Design review of the part built by this model. Coordinates are the model's own, in mm. Face numbers are marked on the shaded views. A direction names the side the tool comes from. Round coordinates to 2 decimals unless told otherwise and drop trailing zeros. Loops run counter-clockwise (first coordinate to the right, second up) from the corner with the lowest first, then second, coordinate; pieces in that order, holes last. Notation, with made-up numbers: (86, 48) - (110, 48) arc R18 ccw to (110, 55) - close; hole circle Ø1 at (47.5, 18.5). An arc over 180 degrees is marked (long way). Use one line per item in the form item = value. Start each with the question number.
(1) We need section B-B, the plane z = -27. Write out the cut boundary in (x, y), then the cut area to 3 significant figures.
(2) Wall thickness on probe 1 along X at (y, z) = (-49, -25); probe 2 along Y at (x, z) = (0, -1); probe 3 along Z at (x, y) = (10, -38): over which ranges is each line inside the solid? List them lowest first. Write a range as [from, to].
(3) We need section A-A, the plane x = 0. Write out the cut boundary in (y, z).
(4) Machinability: for the marked faces 5 and 6, which of the approach directions +Z, -Z, +X, -X, +Y, -Y give a long, thin tool a straight path to every point of the face, cutting with its end or side? Answer none if there is none.
(5) The part is to be moulded in two halves that separate along X. For the marked faces 1, 2, 3 and 4, say which applies: released by +X, released by -X, zero draft, split by the parting line, or undercut.
(6) We need section D-D, the plane z = -38.5. Write out the cut boundary in (x, y).
(7) We need section C-C, the plane y = -55.5. Write out the cut boundary in (x, z), then the cut area to 3 significant figures.
(8) For pin 1 (12 mm diameter, centred on x = 2, y = -11.5, fed in from -Z); pin 2 (3 mm diameter, centred on x = 0, y = 0, fed in from -Z); pin 3 (9 mm diameter, centred on x = 6.5, z = -21, fed in from +Y), all flat-tipped, find the tip position at first contact; note any pin that passes through.
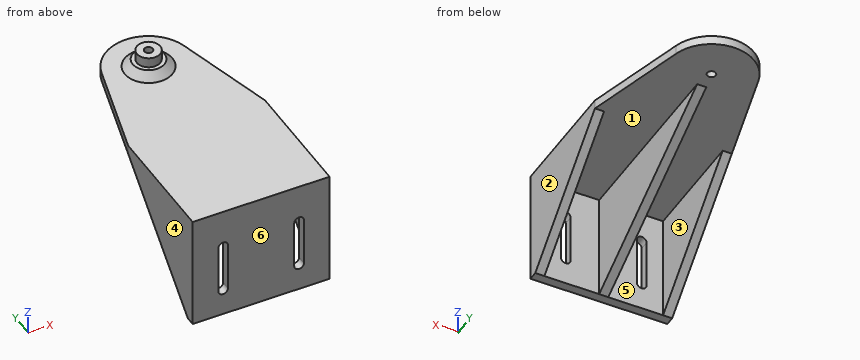
from build123d import *

# Parameters (mm, degrees)
SKETCH_1_R           = 3.85
SKETCH_1_R_2         = 1.4
EXTRUDE_1_DEPTH      = 3.35
SKETCH_3_R           = 7.85
SKETCH_2_R           = 5.2
EXTRUDE_2_DEPTH      = 3
CUT_EXTRUDE_START    = -23.35
SKETCH_7_R           = 1.4
CUT_EXTRUDE_1_DEPTH  = 23.35
SKETCH_11_W          = 44.997612104
SKETCH_11_H          = 3
EXTRUDE_3_DEPTH      = 35
CUT_EXTRUDE_4_DEPTH  = 35
EXTRUDE_4_DEPTH      = 3
EXTRUDE_5_DEPTH      = 1.5
EXTRUDE_5_DEPTH_BACK = 1.5


with BuildPart() as part:
    # 草图1 → 凸台-拉伸1 (new body)
    with BuildSketch(Plane.XY):
        Circle(SKETCH_1_R)
        Circle(SKETCH_1_R_2, mode=Mode.SUBTRACT)
    extrude(amount=-EXTRUDE_1_DEPTH)

    # 草图3 → 放样1 section 0
    with BuildSketch(Plane(origin=(0, 0, -6), x_dir=(-1, 0, 0), z_dir=(0, 0, -1))):
        Circle(SKETCH_3_R)
    # 草图2 → 放样1 section 1
    with BuildSketch(Plane(origin=(0, 0, -3.35), x_dir=(-1, 0, 0), z_dir=(0, 0, -1))):
        Circle(SKETCH_2_R)
    loft()

    # 草图6 → 凸台-拉伸2 (add)
    with BuildSketch(Plane(origin=(0, 0, -6), x_dir=(-1, 0, 0), z_dir=(0, 0, -1))):
        with BuildLine():
            Line((-22.498806052, -29.874841024), (-22.498806052, -69.994841024))
            Line((-22.498806052, -69.994841024), (22.498806052, -69.994841024))
            Line((22.498806052, -69.994841024), (22.498806052, -29.874841024))
            Line((22.498806052, -29.874841024), (13.522961568, 3.623466631))
            ThreePointArc((13.522961568, 3.623466631), (0, 14), (-13.522961568, 3.623466631))
            Line((-13.522961568, 3.623466631), (-22.498806052, -29.874841024))
        make_face()
    extrude(amount=EXTRUDE_2_DEPTH)

    # 草图7 → 切除-拉伸1 (cut)
    with BuildSketch(Plane(origin=(0, 0, -9), x_dir=(-1, 0, 0), z_dir=(0, 0, -1)).offset(CUT_EXTRUDE_START)):
        with Locations(Location((0, 0, 0), (0, 0, 180))):
            Circle(SKETCH_7_R)
    extrude(amount=CUT_EXTRUDE_1_DEPTH, mode=Mode.SUBTRACT)

    # 草图11 → 凸台-拉伸3 (add)
    with BuildSketch(Plane(origin=(0, 0, -9), x_dir=(-1, 0, 0), z_dir=(0, 0, -1))):
        with Locations((0, -68.494841024)):
            Rectangle(SKETCH_11_W, SKETCH_11_H)
    extrude(amount=EXTRUDE_3_DEPTH)

    # 草图14 → 切除-拉伸4 (cut)
    with BuildSketch(Plane(origin=(0, -66.994841024, 0), x_dir=(1, 0, 0), z_dir=(0, 1, 0))):
        with BuildLine():
            Line((14.079686052, 35), (14.079686052, 19))
            ThreePointArc((14.079686052, 19), (12.481386052, 17.4017), (10.883086052, 19))
            Line((10.883086052, 19), (10.883086052, 35))
            ThreePointArc((10.883086052, 35), (12.481386052, 36.5983), (14.079686052, 35))
        make_face()
        with BuildLine():
            ThreePointArc((-10.883086052, 19), (-12.481386052, 17.4017), (-14.079686052, 19))
            Line((-14.079686052, 19), (-14.079686052, 35))
            ThreePointArc((-14.079686052, 35), (-12.481386052, 36.5983), (-10.883086052, 35))
            Line((-10.883086052, 35), (-10.883086052, 19))
        make_face()
    extrude(amount=-CUT_EXTRUDE_4_DEPTH, mode=Mode.SUBTRACT)

    # 草图15 → 凸台-拉伸4 (add)
    with BuildSketch(Plane(origin=(22.498806052, 0, 0), x_dir=(0, 0, -1), z_dir=(1, 0, 0))):
        Polygon((9, -29.874841024), (44, -66.994841024), (44, -69.994841024), (6, -69.994841024), (6, -29.874841024), align=None)
    extrude_4 = extrude(amount=-EXTRUDE_4_DEPTH)

    # 镜向1: 凸台-拉伸4 across plane
    add(extrude_4.mirror(Plane(origin=(0, 0, 0), x_dir=(0, 0, 1), z_dir=(1, 0, 0))))

    # 草图19 → 凸台-拉伸5 (add, two sides: drawn at the far end of the back side and taken through both)
    with BuildSketch(Plane(origin=(0, 0, 0), x_dir=(0, 0, -1), z_dir=(1, 0, 0)).offset(-EXTRUDE_5_DEPTH_BACK)):
        Polygon((44, -66.994841024), (9, -6.021479283), (9, -66.994841024), align=None)
    extrude(amount=EXTRUDE_5_DEPTH + EXTRUDE_5_DEPTH_BACK)


solid = part.part
Data:
q1.outline = (-22.5, -69.99) - (-14.08, -69.99) - (-14.08, -66.99) - (-19.5, -66.99) - (-19.5, -48.97) - (-22.5, -48.97) - close; (-10.88, -69.99) - (10.88, -69.99) - (10.88, -66.99) - (1.5, -66.99) - (1.5, -37.38) - (-1.5, -37.38) - (-1.5, -66.99) - (-10.88, -66.99) - close; (14.08, -69.99) - (22.5, -69.99) - (22.5, -48.97) - (19.5, -48.97) - (19.5, -66.99) - (14.08, -66.99) - close
q1.area = 313 mm^2
q2.probe_1 = [-22.5, -19.5], [-1.5, 1.5], [19.5, 22.5]
q2.probe_2 = [-3.85, -1.4], [1.4, 3.85]
q2.probe_3 = [-9, -6]
q3.outline = (-69.99, -44) - (-66.99, -44) - (-6.02, -9) - (-1.4, -9) - (-1.4, 0) - (-3.85, 0) - (-3.85, -3.35) - (-5.2, -3.35) - (-7.85, -6) - (-69.99, -6) - close; (1.4, -9) - (14, -9) - (14, -6) - (7.85, -6) - (5.2, -3.35) - (3.85, -3.35) - (3.85, 0) - (1.4, 0) - close
q4.face_5 = -Z, +Y
q4.face_6 = +Z, -Z, +X, -X, -Y
q5.face_1 = undercut
q5.face_2 = released by +X
q5.face_3 = undercut
q5.face_4 = released by -X
q6.outline = (-22.5, -69.99) - (22.5, -69.99) - (22.5, -61.16) - (19.5, -61.16) - (19.5, -66.99) - (1.5, -66.99) - (1.5, -57.41) - (-1.5, -57.41) - (-1.5, -66.99) - (-19.5, -66.99) - (-19.5, -61.16) - (-22.5, -61.16) - close
q7.outline = (-22.5, -33.16) - (-19.5, -33.16) - (-19.5, -9) - (-1.5, -9) - (-1.5, -37.4) - (1.5, -37.4) - (1.5, -9) - (19.5, -9) - (19.5, -33.16) - (22.5, -33.16) - (22.5, -6) - (-22.5, -6) - close
q7.area = 365 mm^2
q8.pin_1 = -15.58
q8.pin_2 = -9
q8.pin_3 = -66.99
